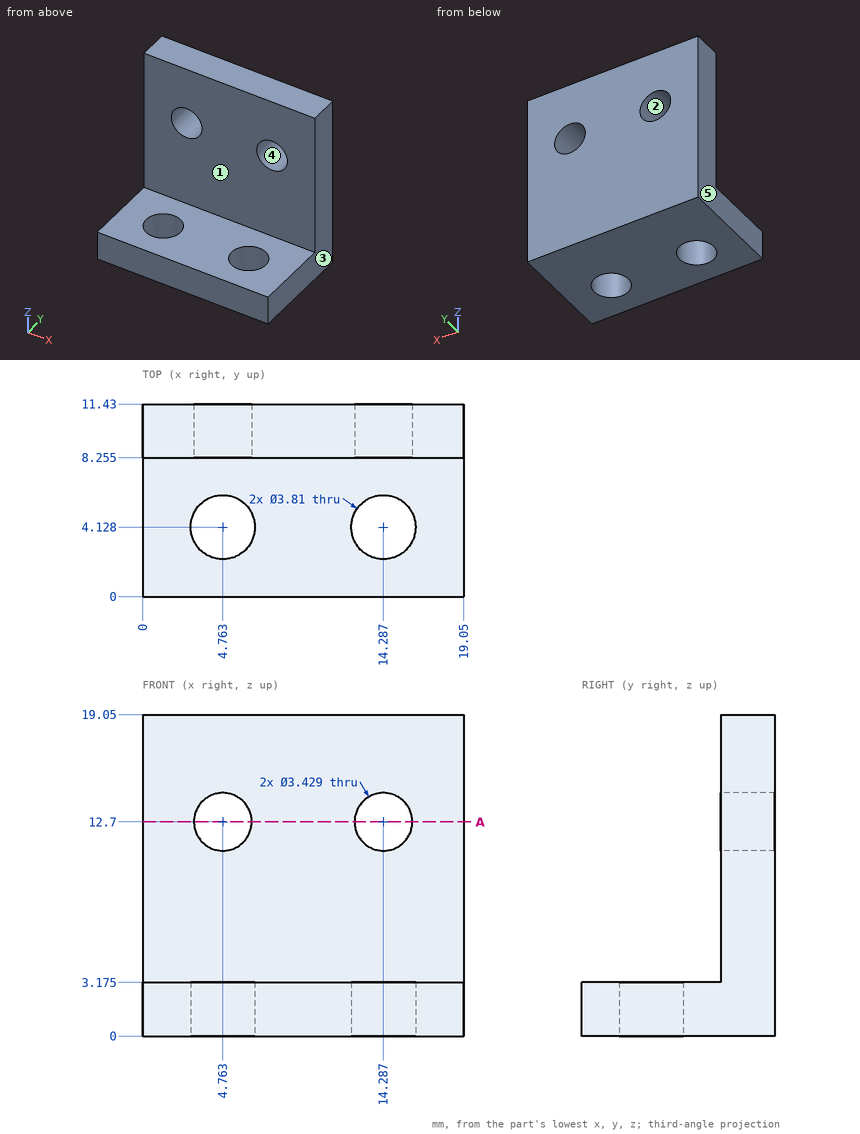
Study the drawing (mm; zero at the part's minimum x, y, z) and answer. A direction names the side the tool comes from. Coordinates: 2 decimals unless noted, no trailing zeros. Write item = value, one per line.
(1) Given pin 1 Ø4 at (x, z) = (10, 6) entering from -Y (1 decimal); pin 2 Ø6 at (x, y) = (14.29, 4.13) entering from +Z (1 decimal); pin 3 Ø3.5 at (x, y) = (4.76, 4.13) entering from -Z, each flat-ended and moving along its own axis, determine where each tip first touches the part or whether it passes through.
From the geometry:
pin_1 = 8.3
pin_2 = 3.2
pin_3 = through
(2) Straight lines are drawn through the part: L1, parallel to X at y = 9.85, z = 12.7; L2, parallel to Y at x = 14.75, z = 4.75 (1 decimal); L3, parallel to Z at x = 11.5, y = 1.5 (1 decimal). For each, find the intervals that lie inside material, in ascending order. Write a range as from..to.
From the geometry:
L1 = 0..3.05, 6.48..12.57, 16..19.05
L2 = 8.3..11.4
L3 = 0..3.2
(3) For a pull along X with two mould halves and no side action, classify the marked faces 3, 4 and 5 as +X half, -X half, draft (parallel to the pull), parting line (faces both ways), or undercut.
From the geometry:
face_3 = +X half
face_4 = undercut
face_5 = -X half
(4) Which of the six approach directions +Z, -Z, +X, -X, +Y, -Y give full straight-line access (tool end or side, diameter ignored) to the marked faces 1 and 2?
From the geometry:
face_1 = +Z, +X, -X, -Y
face_2 = +Y, -Y
(5) Section A-A on z = 12.7 is taken. Count the separate pieces of the cut face and the enclosed holes in it.
From the geometry:
separate_pieces = 3
enclosed_holes = 0
